Can you work these out from the model? Positions are in its coordinate system, mm. Give positions to 0.01 mm unless a question says otherwise; leave off trailing zeros. Order: outer loops, then holes, each group sorted by start corner. A loop starts at its lowest first (then second) coordinate and runs counter-clockwise, first axis right, second up. Notation, with made-up numbers: M 75.5,-4 L 96.5,-4 A5 cw 96.5,5 Z; hole C -9.75,56 d11. An arc over 180 degrees is marked long. Use a Markdown table: item, result. Add a question column.
from build123d import *

# Parameters (mm, degrees)
F0_W     = 6
F0_H     = 6
F0_W_2   = 154.2
F0_H_2   = 10
F0_H_3   = 35
F1_DEPTH = 6.35
F3_D     = 3
F3_DEPTH = 10
F3_TIP   = 0.9012909285
F5_D     = 3
F5_DEPTH = 10
F5_TIP   = 0.9012909285


with BuildPart() as f1:
    # F0 (on Top) → F1 (new body)
    with BuildSketch(Plane.XY):
        with Locations((80.1, -43)):
            Rectangle(F0_W, F0_H)
        with Locations((0, -43)):
            Rectangle(F0_W_2, F0_H)
        with Locations((-80.1, -43)):
            Rectangle(F0_W, F0_H)
        with Locations((80.1, 43)):
            Rectangle(F0_W, F0_H)
        with Locations((0, 43)):
            Rectangle(F0_W_2, F0_H)
        with Locations((-80.1, 43)):
            Rectangle(F0_W, F0_H)
        with Locations((80.1, 0)):
            Rectangle(F0_W, F0_H_2)
        Rectangle(F0_W_2, F0_H_2)
        with Locations((-80.1, 0)):
            Rectangle(F0_W, F0_H_2)
        with Locations((-80.1, 22.5)):
            Rectangle(F0_W, F0_H_3)
        with Locations((-80.1, -22.5)):
            Rectangle(F0_W, F0_H_3)
        with Locations((80.1, 22.5)):
            Rectangle(F0_W, F0_H_3)
        with Locations((80.1, -22.5)):
            Rectangle(F0_W, F0_H_3)
    extrude(amount=F1_DEPTH)

    # F3
    with Locations(Plane(origin=(-83.1, 0, 0), x_dir=(0, -1, 0), z_dir=(-1, 0, 0))):
        with Locations((-42.825, 3.175), (0, 3.175), (42.825, 3.175)):
            Hole(F3_D / 2, depth=F3_DEPTH)
            with Locations((0, 0, -(F3_DEPTH + F3_TIP / 2))):  # 118° drill point
                Cone(0, F3_D / 2, F3_TIP, mode=Mode.SUBTRACT)

    # F5
    with Locations(Plane.YZ.offset(83.1)):
        with Locations((-0.0635787927, 3.175), (-42.825, 3.175), (42.825, 3.175)):
            Hole(F5_D / 2, depth=F5_DEPTH)
            with Locations((0, 0, -(F5_DEPTH + F5_TIP / 2))):  # 118° drill point
                Cone(0, F5_D / 2, F5_TIP, mode=Mode.SUBTRACT)


solid = f1.part
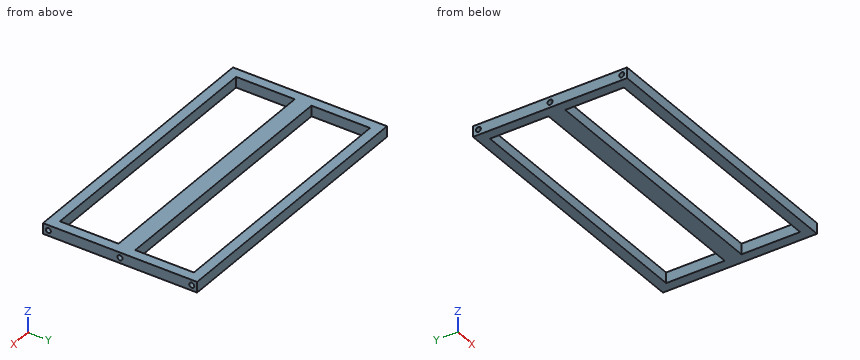
1. If we section it at B-B, the plane y = -25: List the corners of the cut face in (x, z) for me, then the cut area to 3 significant figures.
2. If we section it at A-A, the plane x = -2: List the corners of the cut face in (y, z) for me, then the cut area to 3 significant figures.
3. I need wall thicknesses on L1, parallel to Y at x = -72, z = 4.25; L2, parallel to X at y = 15.5, z = 3.75; L3, parallel to Z at x = -77, y = 0 (3 decimals). Which ranges of each line are inside material? Lowest first, please. Write a range as [from, to].
4. Will these pins go through, and if not, where does the flat tip stop? pin 1 (1.8 mm diameter, centred on y = 0, z = 3.175, fed in from -X); pin 2 (1.8 mm diameter, centred on y = 42.825, z = 3.175, fed in from +X); pin 3 (2.5 mm diameter, centred on y = -42.825, z = 3.175, fed in from +X).
Geometry results:
| question | item | result |
|---|---|---|
| 1 | outline | M -83.1,0 L -77.1,0 L -77.1,6.35 L -83.1,6.35 Z; M 77.1,0 L 83.1,0 L 83.1,6.35 L 77.1,6.35 Z |
| 1 | area | 76.2 mm^2 |
| 2 | outline | M -46,0 L -40,0 L -40,6.35 L -46,6.35 Z; M -5,0 L 5,0 L 5,6.35 L -5,6.35 Z; M 40,0 L 46,0 L 46,6.35 L 40,6.35 Z |
| 2 | area | 140 mm^2 |
| 3 | L1 | y = [-46, -40], [-5, 5], [40, 46] |
| 3 | L2 | x = [-83.1, -77.1], [77.1, 83.1] |
| 3 | L3 | z = [0, 1.675], [4.675, 6.35] |
| 4 | pin 1 | stops at x = -72.74 |
| 4 | pin 2 | stops at x = 72.74 |
| 4 | pin 3 | stops at x = 72.95 |
